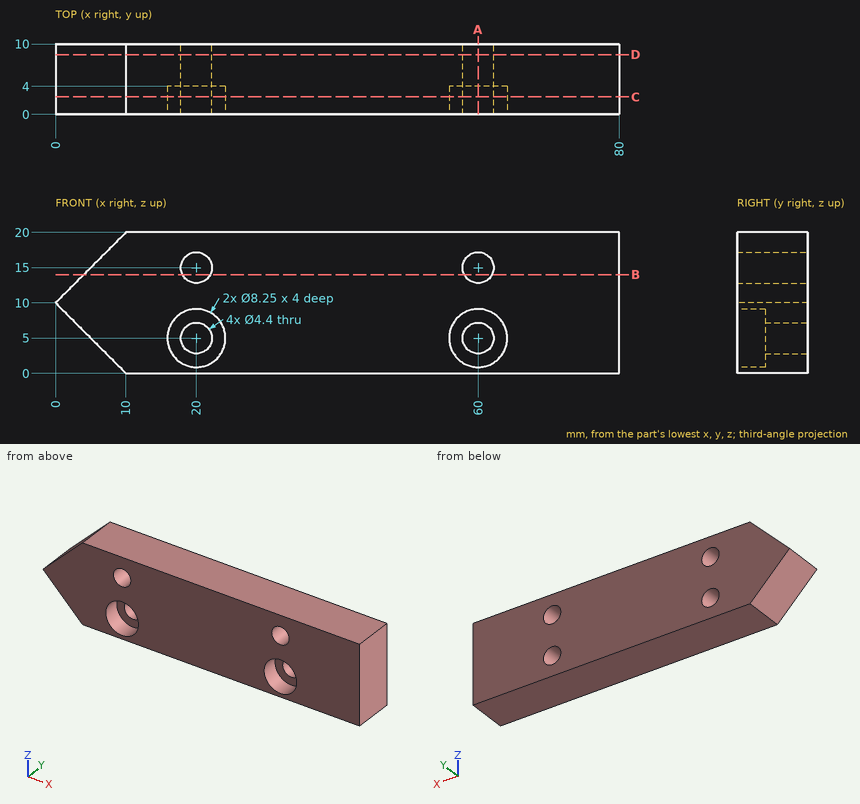
Study the drawing (mm; zero at the part's minimum x, y, z) and answer. Coordinates: 2 decimals unless noted, no trailing zeros. Write each loop counter-clockwise with the first axis right and the second up, starting at its lowest first coordinate (ties: lowest second). Pieces come first, ordered by that corner, then holes. Notation, with made-up numbers: (-17, -22.5) -> (15, -22.5) arc R22 ccw to (15, -11.5) -> close; hole circle Ø6 at (70, 49). An arc over 180 degrees is marked (long way). Write each question's results on one line, items separated by ' | '. Start each with the question number.
1) A cutting plane is placed at B-B (z = 14). Determine the outline of the cut face in (x, y), then the cut area to 3 significant figures.
2) A cutting plane is placed at A-A (x = 60). Determine the outline of the cut face in (y, z) (3 decimals).
3) A cutting plane is placed at D-D (y = 8.5). Determine the outline of the cut face in (x, z).
4) A cutting plane is placed at C-C (y = 2.5). Determine the outline of the cut face in (x, z) (3 decimals), then the cut area to 3 significant figures.
5) Flat-ended cylindrical pins translate along their axes: pin 1 Ø4 at (x, z) = (18, 3.5) entering from -Y; pin 2 Ø6.5 at (x, z) = (60, 5) entering from -Y; pin 3 Ø1.5 at (y, z) = (5.5, 16) entering from -X. Find the tip coordinate at first contact, or state that the pin passes through.
6) Straight lines are drawn through the part: probe 1 along Z at (x, y) = (20, 5.8); probe 2 along Z at (x, y) = (60, 2.85) (3 decimals); probe 3 along X at (y, z) = (1.5, 5.5). For each, find the intervals that lie inside material, in ascending order.
Values follow:
1) outline: (4, 0) -> (18.04, 0) -> (18.04, 10) -> (4, 10) -> close; (21.96, 0) -> (58.04, 0) -> (58.04, 10) -> (21.96, 10) -> close; (61.96, 0) -> (80, 0) -> (80, 10) -> (61.96, 10) -> close | area: 682 mm²
2) outline: (0, 0) -> (10, 0) -> (10, 2.8) -> (4, 2.8) -> (4, 0.875) -> (0, 0.875) -> close; (0, 9.125) -> (4, 9.125) -> (4, 7.2) -> (10, 7.2) -> (10, 12.8) -> (0, 12.8) -> close; (0, 17.2) -> (10, 17.2) -> (10, 20) -> (0, 20) -> close
3) outline: (0, 10) -> (10, 0) -> (80, 0) -> (80, 20) -> (10, 20) -> close; hole circle Ø4.4 at (20, 5); hole circle Ø4.4 at (20, 15); hole circle Ø4.4 at (60, 5); hole circle Ø4.4 at (60, 15)
4) outline: (0, 10) -> (10, 0) -> (80, 0) -> (80, 20) -> (10, 20) -> close; hole circle Ø8.25 at (20, 5); hole circle Ø4.4 at (20, 15); hole circle Ø8.25 at (60, 5); hole circle Ø4.4 at (60, 15) | area: 1,360 mm²
5) pin 1: y = 0 | pin 2: y = 4 | pin 3: x = 5.25
6) probe 1: 0 to 2.8, 7.2 to 12.8, 17.2 to 20 | probe 2: 0 to 0.875, 9.125 to 12.8, 17.2 to 20 | probe 3: 4.5 to 15.91, 24.09 to 55.91, 64.09 to 80
